Geometry check sheet. Reference: the model listing, model coordinates, mm. Face numbers are marked on the shaded views. Coordinates: 2 decimals unless noted, no trailing zeros. Write each loop counter-clockwise with the first axis right and the second up, starting at its lowest first coordinate (ties: lowest second). Pieces come first, ordered by that corner, then holes. Notation, with made-up numbers: M 5.5,81.25 L 32.5,81.25 A27 cw 32.5,115.25 Z; hole C 44.25,18.25 d9. An arc over 180 degrees is marked long. Write item = value, one per line. Start each with the question number.
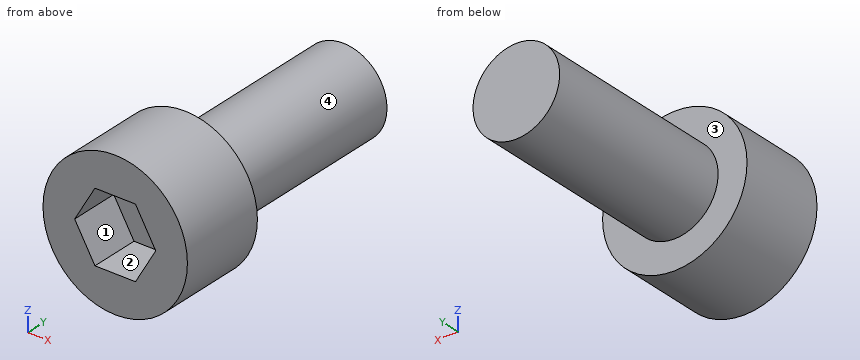
```python
from build123d import *

# Parameters (mm, degrees)
SKETCH1_R           = 2.8575
BOSS_EXTRUDE1_DEPTH = 3.5052
CUT_EXTRUDE1_DEPTH  = 1.9558
SKETCH3_R           = 1.7145
BOSS_EXTRUDE2_DEPTH = 7.9375


with BuildPart() as part:
    # Sketch1 → Boss-Extrude1 (new body)
    with BuildSketch(Plane(origin=(0, 0, 0), x_dir=(1, 0, 0), z_dir=(0, 1, 0))):
        Circle(SKETCH1_R)
    extrude(amount=BOSS_EXTRUDE1_DEPTH)

    # Sketch2 → Cut-Extrude1 (cut)
    with BuildSketch(Plane.XZ):
        Polygon((1.603951217, 0), (0.801975608, 1.3890625), (-0.801975608, 1.3890625), (-1.603951217, 0), (-0.801975608, -1.3890625), (0.801975608, -1.3890625), align=None)
    extrude(amount=-CUT_EXTRUDE1_DEPTH, mode=Mode.SUBTRACT)

    # Sketch3 → Boss-Extrude2 (add)
    with BuildSketch(Plane(origin=(0, 3.5052, 0), x_dir=(1, 0, 0), z_dir=(0, 1, 0))):
        Circle(SKETCH3_R)
    extrude(amount=BOSS_EXTRUDE2_DEPTH)


solid = part.part
```
Q1. Scan lines: L1, parallel to Y at x = -1.7, z = 1.75; L2, parallel to Z at x = -0.6, y = 4; L3, parallel to Z at x = -0.05, y = 5. Record each from-to range of solid material in increasing order.
Q2. Cross-section at B-B on x = 0. Enter the section's corners in (y, z).
Q3. Cross-section at D-D on y = 5. Enter the section's corners in (x, z), and give its area (3 significant figures).
Q4. Gauge pin test, flat ends, axial feed: pin 1 (2 mm diameter, centred on x = 0, y = 8.5, fed in from -Z); pin 2 (0.5 mm diameter, centred on x = 0.5, y = 0.5, fed in from +Z). Record the tip position at first contact, or that the pin passes through.
Q5. Draft check along Z on the marked faces 1, 2, 3 and 4. Enter one of: pulls with the +Z half, pulls with the -Z half, needs draft (parallel to the pull), parting line crosses it, or undercut.
Q6. Cross-section at A-A on y = 1.5. Enter the section's corners in (x, z) (1 decimal).
Q7. Cross-section at C-C on z = 0.5. Enter the section's corners in (x, y).
Values found:
q1.L1 = 0 to 3.51
q1.L2 = -1.61 to 1.61
q1.L3 = -1.71 to 1.71
q2.outline = M 0,-2.86 L 3.51,-2.86 L 3.51,-1.71 L 11.44,-1.71 L 11.44,1.71 L 3.51,1.71 L 3.51,2.86 L 0,2.86 L 0,1.39 L 1.96,1.39 L 1.96,-1.39 L 0,-1.39 Z
q3.outline = C 0,0 d3.43
q3.area = 9.23 mm²
q4.pin_1 = -1.71
q4.pin_2 = 2.85
q5.face_1 = undercut
q5.face_2 = undercut
q5.face_3 = needs draft
q5.face_4 = parting line crosses it
q6.outline = C 0,0 d5.7; hole M -1.6,0 L -0.8,-1.4 L 0.8,-1.4 L 1.6,0 L 0.8,1.4 L -0.8,1.4 Z
q7.outline = M -2.81,0 L -1.32,0 L -1.32,1.96 L 1.32,1.96 L 1.32,0 L 2.81,0 L 2.81,3.51 L 1.64,3.51 L 1.64,11.44 L -1.64,11.44 L -1.64,3.51 L -2.81,3.51 Z
